```python
from build123d import *

# Parameters (mm, degrees)
SKETCH1_R           = 3.5
BOSS_EXTRUDE1_DEPTH = 5
SKETCH2_R           = 2.5
BOSS_EXTRUDE2_DEPTH = 25
CUT_EXTRUDE1_DEPTH  = 2
CHAMFER1_SIZE       = 0.25
FILLET1_R           = 0.2


with BuildPart() as part:
    # Sketch1 → Boss-Extrude1 (new body)
    with BuildSketch(Plane(origin=(0, 0, 0), x_dir=(1, 0, 0), z_dir=(0, 1, 0))):
        with Locations(Location((0, 0, 0), (0, 0, 270))):
            Circle(SKETCH1_R)
    extrude(amount=BOSS_EXTRUDE1_DEPTH)

    # Sketch2 → Boss-Extrude2 (add)
    with BuildSketch(Plane(origin=(0, 5, 0), x_dir=(1, 0, 0), z_dir=(0, 1, 0))):
        with Locations(Location((0, 0, 0), (0, 0, 270))):
            Circle(SKETCH2_R)
    extrude(amount=BOSS_EXTRUDE2_DEPTH)

    # Sketch3 → Cut-Extrude1 (cut)
    with BuildSketch(Plane.XZ):
        Polygon((0, 2), (-1.732050808, 1), (-1.732050808, -1), (0, -2), (1.732050808, -1), (1.732050808, 1), align=None)
    extrude(amount=-CUT_EXTRUDE1_DEPTH, mode=Mode.SUBTRACT)

    # Chamfer1
    chamfer1_edges = [part.edges().sort_by_distance(p)[0] for p in [
        (0.866025404, 0, 1.5),
        (-0.866025404, 0, 1.5),
        (-1.732050808, 0, 0),
        (-0.866025404, 0, -1.5),
        (0.866025404, 0, -1.5),
        (1.732050808, 0, 0),
    ]]
    chamfer(chamfer1_edges, length=CHAMFER1_SIZE)

    # Fillet1
    fillet1_edges = [part.edges().sort_by_distance(p)[0] for p in [
        (0, 0, -3.5),
    ]]
    fillet(fillet1_edges, radius=FILLET1_R)


solid = part.part
```
CAD build for the part. Positions are in the model's coordinates, mm. A direction names the side the tool comes from. Round coordinates to 2 decimals unless told otherwise and drop trailing zeros. Write each loop counter-clockwise with the first axis right and the second up, starting at its lowest first coordinate (ties: lowest second). Pieces come first, ordered by that corner, then holes. Notation, with made-up numbers: (-33, -30.5) - (11, -30.5) arc R22 cw to (11, -17.5) - close; hole circle Ø10 at (1.5, 85.25). An arc over 180 degrees is marked (long way). Return JSON: item names as keys, results as strings. Group by question number.
Item 1: Flat gauge pins, fed straight in: pin 1 Ø1.5 at (x, y) = (2, 3) entering from +Z; pin 2 Ø1 at (y, z) = (4, -2.5) entering from -X; pin 3 Ø1 at (x, y) = (-1, 26.5) entering from +Z. Where does each tip first touch, or does it go through?
Item 2: Probe probe 1 along Y at (x, z) = (0.75, 1); probe 2 along X at (y, z) = (23.5, -1); probe 3 along Z at (x, y) = (1.5, 9.75). List the from-to ranges inside material, lowest first.
Item 3: Mould opens along X. For faces 1 (the face through (-1.732, 1, 0)), 2 (the face through (-1, 0, -2)), 3 (the face through (0, 2, 0)), 4 (the face through (-2.44, 17.32, -0.54)) say: +X half, -X half, draft (parallel to the pull), parting line (faces both ways), or undercut.
Item 4: Band-saw the part on A-A on z = 0. List the corners of the cut face in (x, y).
Item 5: 3-axis set-ups, long thin cutter, end or side, ignore diameter. For faces 5 (the face through (0, 30, 0)), 6 (the face through (-0.91, 0.13, 1.61)), 7 (the face through (-2, 5, 2)): which of +Z, -Z, +X, -X, +Y, -Y reach the whole face in a straight line?
Item 6: Band-saw the part on B-B on y = 18. List the corners of the cut face in (x, z).
Resolved:
{
 "1": {"pin 1": "stops at z = 3.27", "pin 2": "stops at x = -2.87", "pin 3": "stops at z = 2.45"},
 "2": {"probe 1": "y = 2 to 30", "probe 2": "x = -2.29 to 2.29", "probe 3": "z = -2 to 2"},
 "3": {"face 1": "undercut", "face 2": "draft", "face 3": "undercut", "face 4": "parting line"},
 "4": {"outline": "(-3.5, 0.2) arc R0.2 ccw to (-3.3, 0) - (-1.98, 0) - (-1.73, 0.25) - (-1.73, 2) - (1.73, 2) - (1.73, 0.25) - (1.98, 0) - (3.3, 0) arc R0.2 ccw to (3.5, 0.2) - (3.5, 5) - (2.5, 5) - (2.5, 30) - (-2.5, 30) - (-2.5, 5) - (-3.5, 5) - close"},
 "5": {"face 5": "+Z, -Z, +X, -X, +Y", "face 6": "-Y", "face 7": "+Y"},
 "6": {"outline": "circle Ø5 at (0, 0)"}
}
